Here's how the part is built. I have some questions about the finished solid (model axes, mm). Face numbers are marked on the shaded views. A direction names the side the tool comes from. Coordinates: 2 decimals unless noted, no trailing zeros. Order: outer loops, then holes, each group sorted by start corner. A loop starts at its lowest first (then second) coordinate and runs counter-clockwise, first axis right, second up.
```python
from build123d import *

# Parameters (mm, degrees)
F1_DEPTH = 63.5
F0_W     = 25.2919347882
F0_H     = 19.05
F2_DEPTH = 25.4
F3_DEPTH = 8.5725


with BuildPart() as f1:
    # F0 (on Front) → F1 (new body, symmetric)
    with BuildSketch(Plane.XZ):
        Polygon((22.225, 9.525), (-41.275, 9.525), (-41.275, -9.525), (41.275, -9.525), (41.275, 9.525), align=None)
    extrude(amount=F1_DEPTH, both=True)

    # F0 (on Front) → F2 (join, symmetric)
    with BuildSketch(Plane.XZ):
        with BuildLine():
            Line((22.225, 27.0002), (22.225, 9.525))
            Line((22.225, 9.525), (41.275, 9.525))
            Line((41.275, 9.525), (41.275, 27.0002))
            ThreePointArc((41.275, 27.0002), (45.9246798487, 38.2255201513), (57.15, 42.8752))
            Line((57.15, 42.8752), (60.4330652118, 42.8752))
            Line((60.4330652118, 42.8752), (60.4330652118, 61.9252))
            Line((60.4330652118, 61.9252), (57.15, 61.9252))
            add(Edge.make_bspline(
                [(55.1864649446, 61.8699598943), (55.8526018083, 61.9015411095), (56.5073505407, 61.9200895907), (57.15, 61.9252)],
                knots=[109.3417513955, 109.3417513955, 109.3417513955, 109.3417513955, 111.5045361635, 111.5045361635, 111.5045361635, 111.5045361635], degree=3))
            ThreePointArc((55.1864649446, 61.8699598943), (31.7695736165, 50.9916480929), (22.225, 27.0002))
        make_face()
        with Locations((73.0790326059, 52.4002)):
            Rectangle(F0_W, F0_H)
    extrude(amount=F2_DEPTH, both=True)

    # F0 (on Front) → F3 (join, symmetric)
    with BuildSketch(Plane.XZ):
        with BuildLine():
            add(Edge.make_bspline(
                [(-41.275, 9.525), (-41.275, 25.3662331122), (21.509248225, 60.2733399101), (55.1864649446, 61.8699598943)],
                knots=[0, 0, 0, 0, 109.3417513955, 109.3417513955, 109.3417513955, 109.3417513955], degree=3))
            Line((-41.275, 9.525), (22.225, 9.525))
            Line((22.225, 9.525), (22.225, 27.0002))
            ThreePointArc((22.225, 27.0002), (31.7695736165, 50.9916480929), (55.1864649446, 61.8699598943))
        make_face()
    extrude(amount=F3_DEPTH, both=True)


solid = f1.part
```
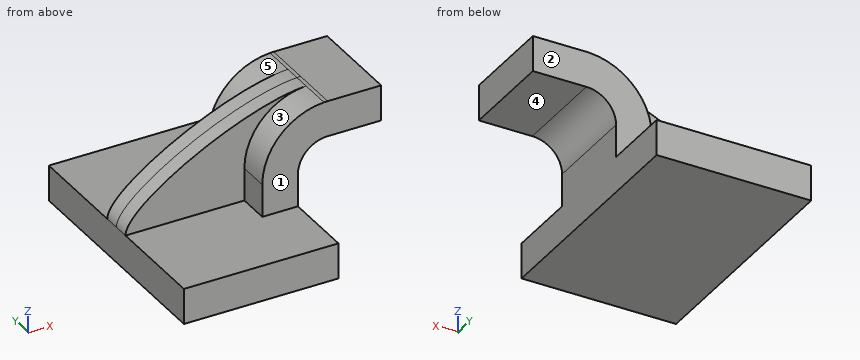
Q1. I need wall thicknesses on L1, parallel to Z at x = -34, y = -49 (3 decimals); L2, parallel to Y at x = 46, z = 44; L3, parallel to X at y = 35.5, z = -4 (3 decimals). Which ranges of each line are inside material? Lowest first, please.
Q2. If we section it at B-B on z = 0: Write out the boundary of the cut face in (x, y) (3 decimals), then the cut area to 3 significant figures.
Q3. For the marked faces 1, 2, 3, 4 and 5, which set-ups out of +Z, -Z, +X, -X, +Y, -Y let a thin tool reach every point of the face, with its end or its side?
Q4. If we section it at A-A on x = 76: Write out the boundary of the cut face in (y, z), then the cut area to 3 significant figures.
Q5. Will these pins go through, and if not, where does the flat tip stop? pin 1 (1.5 mm diameter, centred on x = 44, y = 16.5, fed in from -Z); pin 2 (5 mm diameter, centred on y = 20.5, z = 17.5, fed in from -X) (3 decimals); pin 3 (16.5 mm diameter, centred on x = 2, y = -33.5, fed in from +Z) (3 decimals).
Reply:
1. L1: z = -9.525 to 9.525
1. L2: y = -25.4 to 25.4
1. L3: x = -41.275 to 41.275
2. outline: (-41.275, -63.5) - (41.275, -63.5) - (41.275, 63.5) - (-41.275, 63.5) - close
2. area: 10,500 mm2
3. face 1: +Z, +X, -X, -Y
3. face 2: +Z, +X, -X, +Y
3. face 3: +Z, -X, -Y
3. face 4: -Z, +X, +Y, -Y
3. face 5: +Z, -X, +Y
4. outline: (-25.4, 42.88) - (25.4, 42.88) - (25.4, 61.93) - (-25.4, 61.93) - close
4. area: 968 mm2
5. pin 1: stops at z = 34.67
5. pin 2: stops at x = 22.225
5. pin 3: stops at z = 9.525
